```python
from build123d import *

# Parameters (mm, degrees)
SKETCH1_W           = 139.7
SKETCH1_H           = 88.9
SKETCH1_R           = 1.4732
BOSS_EXTRUDE1_DEPTH = 2.54
FILLET1_R           = 6.35


with BuildPart() as part:
    # Sketch1 → Boss-Extrude1 (new body)
    with BuildSketch(Plane(origin=(0, 0, 0), x_dir=(1, 0, 0), z_dir=(0, 1, 0))):
        with Locations((69.85, -44.45)):
            Rectangle(SKETCH1_W, SKETCH1_H)
        with Locations(Location((34.85, -9.45, 0), (0, 0, 270))):
            Circle(SKETCH1_R, mode=Mode.SUBTRACT)
        with Locations(Location((6.35, -6.35, 0), (0, 0, 270))):
            Circle(SKETCH1_R, mode=Mode.SUBTRACT)
        with Locations(Location((6.35, -19.05, 0), (0, 0, 270))):
            Circle(SKETCH1_R, mode=Mode.SUBTRACT)
        with Locations(Location((6.35, -31.75, 0), (0, 0, 270))):
            Circle(SKETCH1_R, mode=Mode.SUBTRACT)
        with Locations(Location((6.35, -44.45, 0), (0, 0, 270))):
            Circle(SKETCH1_R, mode=Mode.SUBTRACT)
        with Locations(Location((6.35, -57.15, 0), (0, 0, 270))):
            Circle(SKETCH1_R, mode=Mode.SUBTRACT)
        with Locations(Location((6.35, -69.85, 0), (0, 0, 270))):
            Circle(SKETCH1_R, mode=Mode.SUBTRACT)
        with Locations(Location((6.35, -82.55, 0), (0, 0, 270))):
            Circle(SKETCH1_R, mode=Mode.SUBTRACT)
        with Locations(Location((104.85, -9.45, 0), (0, 0, 270))):
            Circle(SKETCH1_R, mode=Mode.SUBTRACT)
        with Locations(Location((104.85, -79.45, 0), (0, 0, 270))):
            Circle(SKETCH1_R, mode=Mode.SUBTRACT)
        with Locations(Location((34.85, -79.45, 0), (0, 0, 270))):
            Circle(SKETCH1_R, mode=Mode.SUBTRACT)
        with Locations(Location((133.35, -82.55, 0), (0, 0, 90))):
            Circle(SKETCH1_R, mode=Mode.SUBTRACT)
        with Locations(Location((133.35, -69.85, 0), (0, 0, 90))):
            Circle(SKETCH1_R, mode=Mode.SUBTRACT)
        with Locations(Location((133.35, -57.15, 0), (0, 0, 90))):
            Circle(SKETCH1_R, mode=Mode.SUBTRACT)
        with Locations(Location((133.35, -44.45, 0), (0, 0, 90))):
            Circle(SKETCH1_R, mode=Mode.SUBTRACT)
        with Locations(Location((133.35, -31.75, 0), (0, 0, 90))):
            Circle(SKETCH1_R, mode=Mode.SUBTRACT)
        with Locations(Location((133.35, -19.05, 0), (0, 0, 90))):
            Circle(SKETCH1_R, mode=Mode.SUBTRACT)
        with Locations(Location((133.35, -6.35, 0), (0, 0, 90))):
            Circle(SKETCH1_R, mode=Mode.SUBTRACT)
        with Locations(Location((19.05, -44.45, 0), (0, 0, 270))):
            Circle(SKETCH1_R, mode=Mode.SUBTRACT)
        with Locations(Location((120.65, -44.45, 0), (0, 0, 270))):
            Circle(SKETCH1_R, mode=Mode.SUBTRACT)
    extrude(amount=BOSS_EXTRUDE1_DEPTH)

    # Fillet1
    fillet1_edges = [part.edges().sort_by_distance(p)[0] for p in [
        (0, 1.27, 0),
        (139.7, 1.27, 0),
        (139.7, 1.27, 88.9),
        (0, 1.27, 88.9),
    ]]
    fillet(fillet1_edges, radius=FILLET1_R)


solid = part.part
```
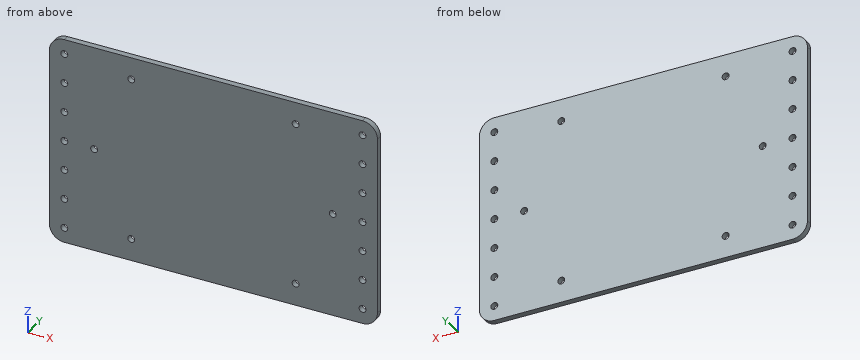
The listing builds one solid part. Answer for the finished solid, in the listing's coordinates (mm). Round coordinates to 2 decimals unless told otherwise and drop trailing zeros. Write each loop counter-clockwise with the first axis right and the second up, starting at its lowest first coordinate (ties: lowest second). Pieces come first, ordered by that corner, then holes. Notation, with made-up numbers: (9.5, 76.25) -> (23.5, 76.25) arc R24 ccw to (23.5, 87.25) -> close; hole circle Ø3 at (-11, 71). An arc over 180 degrees is marked (long way). Answer as a JSON object with one key per item and string values. Group by question number.
Q1. Section B-B (x = 19.05) is taken. Write down the section's boundary in (y, z), plus the area to 3 significant figures.
Q2. Section D-D (x = 34.85) is taken. Write down the section's boundary in (y, z).
Q3. Straight lines are drawn through the part: line 1 along X through (y, z) = (1.4, 44.45); line 2 along X through (y, z) = (0.75, 70); line 3 along X through (y, z) = (1.05, 9.45). For each, find the intervals that lie inside material, in ascending order.
Q4. Section C-C (z = 44.45) is taken. Write down the section's boundary in (x, y).
Q5. Section A-A (z = 19.05) is taken. Write down the section's boundary in (x, y), plus the area to 3 significant figures.
Check values:
{
 "1": {"outline": "(0, 0) -> (2.54, 0) -> (2.54, 42.98) -> (0, 42.98) -> close; (0, 45.92) -> (2.54, 45.92) -> (2.54, 88.9) -> (0, 88.9) -> close", "area": "218 mm^2"},
 "2": {"outline": "(0, 0) -> (2.54, 0) -> (2.54, 7.98) -> (0, 7.98) -> close; (0, 10.92) -> (2.54, 10.92) -> (2.54, 77.98) -> (0, 77.98) -> close; (0, 80.92) -> (2.54, 80.92) -> (2.54, 88.9) -> (0, 88.9) -> close"},
 "3": {"line 1": "0 to 4.88, 7.82 to 17.58, 20.52 to 119.18, 122.12 to 131.88, 134.82 to 139.7", "line 2": "0 to 4.88, 7.82 to 131.88, 134.82 to 139.7", "line 3": "0 to 33.38, 36.32 to 103.38, 106.32 to 139.7"},
 "4": {"outline": "(0, 0) -> (4.88, 0) -> (4.88, 2.54) -> (0, 2.54) -> close; (7.82, 0) -> (17.58, 0) -> (17.58, 2.54) -> (7.82, 2.54) -> close; (20.52, 0) -> (119.18, 0) -> (119.18, 2.54) -> (20.52, 2.54) -> close; (122.12, 0) -> (131.88, 0) -> (131.88, 2.54) -> (122.12, 2.54) -> close; (134.82, 0) -> (139.7, 0) -> (139.7, 2.54) -> (134.82, 2.54) -> close"},
 "5": {"outline": "(0, 0) -> (4.88, 0) -> (4.88, 2.54) -> (0, 2.54) -> close; (7.82, 0) -> (131.88, 0) -> (131.88, 2.54) -> (7.82, 2.54) -> close; (134.82, 0) -> (139.7, 0) -> (139.7, 2.54) -> (134.82, 2.54) -> close", "area": "340 mm^2"}
}
